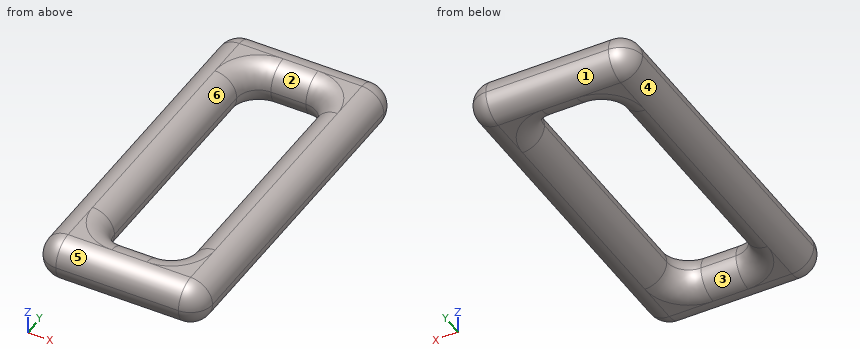
```python
from build123d import *

# Parameters (mm, degrees)
SKETCH1_W           = 190
SKETCH1_H           = 400
SKETCH1_W_2         = 90
SKETCH1_H_2         = 300
BOSS_EXTRUDE1_DEPTH = 25
FILLET1_R           = 25


with BuildPart() as part:
    # Sketch1 → Boss-Extrude1 (new, symmetric)
    with BuildSketch(Plane.XY):
        with Locations((0, -175)):
            Rectangle(SKETCH1_W, SKETCH1_H)
        with Locations((0, -175)):
            Rectangle(SKETCH1_W_2, SKETCH1_H_2, mode=Mode.SUBTRACT)
    extrude(amount=BOSS_EXTRUDE1_DEPTH, both=True)

    # Fillet1
    fillet1_edges = [part.edges().sort_by_distance(p)[0] for p in [
        (95, -175, 25),
        (0, 25, 25),
        (-45, -175, -25),
        (-45, -25, 0),
        (0, -325, -25),
        (-45, -325, 0),
        (45, -175, -25),
        (45, -325, 0),
        (0, -25, -25),
        (45, -25, 0),
        (-45, -175, 25),
        (0, -325, 25),
        (45, -175, 25),
        (0, -25, 25),
        (-95, -175, 25),
        (0, 25, -25),
        (95, -175, -25),
        (0, -375, -25),
        (-95, -175, -25),
        (0, -375, 25),
        (-95, 25, 0),
        (95, 25, 0),
        (95, -375, 0),
        (-95, -375, 0),
    ]]
    fillet(fillet1_edges, radius=FILLET1_R - 0.0001)  # a hair under: the kernel refuses the full size


solid = part.part
```
Geometry check sheet. Reference: the model listing, model coordinates, mm. Face numbers are marked on the shaded views. A direction names the side the tool comes from. Round coordinates to 2 decimals unless told otherwise and drop trailing zeros. Loops run counter-clockwise (first coordinate to the right, second up) from the corner with the lowest first, then second, coordinate; pieces in that order, holes last. Notation, with made-up numbers: (-16.75, -39.75) - (29.25, -39.75) arc R20 ccw to (29.25, -2.75) - close; hole circle Ø5 at (38, -26). An arc over 180 degrees is marked (long way). Use a Markdown table: item, result.
Q1. Go/stop test with flat-tipped pins: P1, Ø1, axis at y = -87, z = 8, coming from the -X side; P2, Ø2, axis at x = 47.5, y = -334.5, coming from the -Z side; P3, Ø10, axis at x = -51, y = -154.5, coming from the +Z side. Record where each tip stops, or that it passes through.
Solutions:
| item | result |
|---|---|
| P1 | stops at x = -93.85 |
| P2 | stops at z = -24.52 |
| P3 | stops at z = 20.71 |
Q2. Material ranges on line 1 (X direction, y = -211.5, z = 0.5) (3 decimals); line 2 (Y direction, x = 19.5, z = 21); line 3 (X direction, y = -271, z = 4.5), recorded low to high.
Solutions:
| item | result |
|---|---|
| line 1 | x = -94.995 to -45.005, 45.005 to 94.995 |
| line 2 | y = -363.56 to -336.44, -13.56 to 13.56 |
| line 3 | x = -94.59 to -45.41, 45.41 to 94.59 |
Q3. Access from +Z, -Z, +X, -X, +Y, -Y to the whole of each face (thin tool, end or side, straight path). Record for the marked faces 1, 2 and 3.
Solutions:
| item | result |
|---|---|
| face 1 | -Z, +X, -X, +Y |
| face 2 | +Z |
| face 3 | -Z |
Q4. Draft check along X on the marked faces 4, 5 and 6. Enter one of: released by +X, released by -X, zero draft, split by the parting line, or undercut.
Solutions:
| item | result |
|---|---|
| face 4 | released by -X |
| face 5 | zero draft |
| face 6 | undercut |
Q5. Cross-section at C-C on z = -11. Record the cut outline in (x, y), plus the area to 3 significant figures.
Solutions:
| item | result |
|---|---|
| outline | (-92.45, -350) arc R22.45 ccw to (-70, -372.45) - (70, -372.45) arc R22.45 ccw to (92.45, -350) - (92.45, 0) arc R22.45 ccw to (70, 22.45) - (-70, 22.45) arc R22.45 ccw to (-92.45, 0) - close; hole (-47.55, -300) arc R27.55 ccw to (-20, -327.55) - (20, -327.55) arc R27.55 ccw to (47.55, -300) - (47.55, -50) arc R27.55 ccw to (20, -22.45) - (-20, -22.45) arc R27.55 ccw to (-47.55, -50) - close |
| area | 44,200 mm2 |
